Verification items for the finished model (mm, model axes). Face numbers are marked on the shaded views. A direction names the side the tool comes from. Coordinates: 2 decimals unless noted, no trailing zeros. Write each loop counter-clockwise with the first axis right and the second up, starting at its lowest first coordinate (ties: lowest second). Pieces come first, ordered by that corner, then holes. Notation, with made-up numbers: (37.25, -6) -> (85.25, -6) arc R14 ccw to (85.25, 8) -> close; hole circle Ø1 at (44.25, -24.5). An arc over 180 degrees is marked (long way). Use CSV: the item, a comma, the result in double quotes.
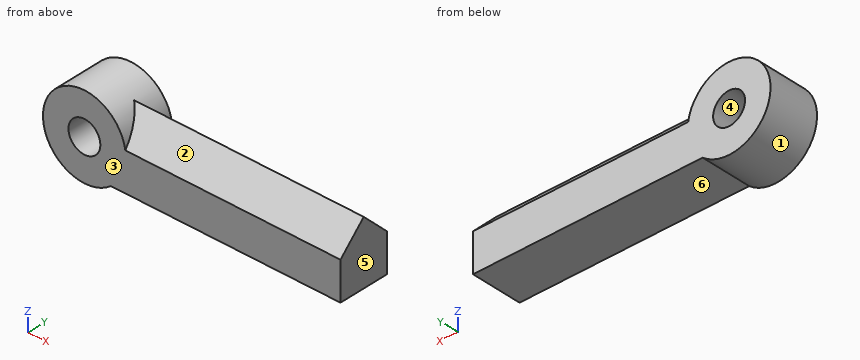
```python
from build123d import *

# Parameters (mm, degrees)
CROQUIS1_R              = 3.25
CROQUIS1_R_2            = 1.25
SALIENTE_EXTRUIR1_DEPTH = 4
CROQUIS2_W              = 18
CROQUIS2_H              = 5
SALIENTE_EXTRUIR2_DEPTH = 4
CHAFL_N1_SIZE           = 2


with BuildPart() as part:
    # Croquis1 → Saliente-Extruir1 (new body)
    with BuildSketch(Plane(origin=(0, 0, 0), x_dir=(1, 0, 0), z_dir=(0, 1, 0))):
        with Locations(Location((0, 0, 0), (0, 0, 270))):
            Circle(CROQUIS1_R)
        with Locations(Location((0, 0, 0), (0, 0, 270))):
            Circle(CROQUIS1_R_2, mode=Mode.SUBTRACT)
    extrude(amount=SALIENTE_EXTRUIR1_DEPTH)

    # Croquis2 → Saliente-Extruir2 (add)
    with BuildSketch(Plane(origin=(0, 4, 0), x_dir=(1, 0, 0), z_dir=(0, 1, 0))):
        with Locations((11.076655966, 0)):
            Rectangle(CROQUIS2_W, CROQUIS2_H)
    extrude(amount=-SALIENTE_EXTRUIR2_DEPTH)

    # Chaflán1
    chafl_n1_edges = [part.edges().sort_by_distance(p)[0] for p in [
        (11.076655966, 4, 2.5),
        (11.076655966, 0, 2.5),
    ]]
    chamfer(chafl_n1_edges, length=CHAFL_N1_SIZE - 0.0001)  # a hair under: the kernel refuses the full size


solid = part.part
```
1) Cross-section at C-C (y = 1.4). Record the boundary of the cut face in (x, z).
Return value:
outline,"(2.08, -2.5) -> (20.08, -2.5) -> (20.08, 1.9) -> (2.64, 1.9) arc R3.25 ccw (long way) to start; hole circle Ø2.5 at (0, 0)"
2) Scan lines: L1, parallel to X at y = 2.2, z = 0; L2, parallel to X at y = 1.55, z = 0.5; L3, parallel to Y at x = 17.75, z = 1.5. Record each from-to range of solid material in increasing order.
Return value:
L1,"-3.25 to -1.25, 1.25 to 20.08"
L2,"-3.21 to -1.15, 1.15 to 20.08"
L3,"1 to 3"
3) Cross-section at B-B (x = 0). Record the boundary of the cut face in (y, z), plus the area to 3 significant figures.
Return value:
outline,"(0, -3.25) -> (4, -3.25) -> (4, -1.25) -> (0, -1.25) -> close; (0, 1.25) -> (4, 1.25) -> (4, 3.25) -> (0, 3.25) -> close"
area,"16.0 mm2"
4) Gauge pin test, flat ends, axial feed: pin 1 (2 mm diameter, centred on x = 14.5, y = 3, fed in from -Z); pin 2 (3 mm diameter, centred on x = 9, z = 2.5, fed in from -Y); pin 3 (1.5 mm diameter, centred on x = 4.5, z = 2, fed in from +Y). Record the tip position at first contact, or that the pin passes through.
Return value:
pin 1,"z = -2.5"
pin 2,"y = 0.5"
pin 3,"y = 3.25"
5) Set-up check for the marked faces 5 and 6: record each of +Z, -Z, +X, -X, +Y, -Y from which the full face is reachable in a straight line by a thin tool's end or side.
Return value:
face 5,"+Z, -Z, +X, +Y, -Y"
face 6,"-Z, +X, +Y, -Y"
6) Mould release check, pull along Z, two halves, no side actions. Record for the marked faces 1, 2, 3 and 4: released by +Z, released by -Z, zero draft, split by the parting line, or undercut.
Return value:
face 1,"split by the parting line"
face 2,"released by +Z"
face 3,"zero draft"
face 4,"undercut"
7) Cross-section at A-A (z = 0). Record the boundary of the cut face in (x, y).
Return value:
outline,"(-3.25, 0) -> (-1.25, 0) -> (-1.25, 4) -> (-3.25, 4) -> close; (1.25, 0) -> (20.08, 0) -> (20.08, 4) -> (1.25, 4) -> close"
